Input: part model. Units: mm. Frame: model coordinates. Face numbers are marked on the shaded views. A direction names the side the tool comes from. Round coordinates to 2 decimals unless told otherwise and drop trailing zeros. Order: outer loops, then holes, each group sorted by start corner. A loop starts at its lowest first (then second) coordinate and runs counter-clockwise, first axis right, second up. Notation, with made-up numbers: (43, 40) -> (57, 40) arc R23 ccw to (57, 57) -> close; hole circle Ø9 at (68.5, -35.75). An arc over 180 degrees is marked (long way). Answer as CSV lines item,"result". Start each with the question number.
1) Section query B-B, the plane z = 43. Output: boundary loops of the cut face in (x, y), and give its area (3 significant figures).
2) Access query for the marked faces 1, 2 and 3. Directions: +Z, -Z, +X, -X, +Y, -Y. A direction counts if a zero-diameter tool reaches every point of the face in a straight line with its end or side. Return the directions, or none.
3) First-contact query: P1, Ø12, axis at x = 79, z = 30, coming from the +Y side; P2, Ø5, axis at y = 70.5, z = 21.5, coming from the +X side. Flat tips, straight axial feed; report the tip coordinate or a pass-through.
4) Line query: L1, parallel to X at y = 37, z = 7; L2, parallel to Y at x = 109.5, z = 47; L3, parallel to Y at x = 33, z = 33.5. Output: solid intervals per line, ascending.
5) Section query A-A, the plane x = 28.5. Output: boundary loops of the cut face in (y, z), and give its area (3 significant figures).
```python
from build123d import *

# Parameters (mm, degrees)
EXTRUDE_1_DEPTH     = 80
SKETCH_2_W          = 10
SKETCH_2_H          = 70
CUT_EXTRUDE_1_DEPTH = 250
SKETCH_3_W          = 70
SKETCH_3_H          = 10
CUT_EXTRUDE_2_DEPTH = 250
SKETCH_4_R          = 2.692710991
CUT_EXTRUDE_3_DEPTH = 10


with BuildPart() as part:
    # Эскиз1 → Бобышка-Вытянуть1 (new body)
    with BuildSketch(Plane.XY):
        Polygon((0, 0), (0, 220), (250, 220), (250, 140), (80, 140), (80, 0), align=None)
    extrude(amount=EXTRUDE_1_DEPTH)

    # Эскиз2 → Вырез-Вытянуть1 (cut)
    with BuildSketch(Plane.XZ):
        with Locations((5, 35)):
            Rectangle(SKETCH_2_W, SKETCH_2_H)
    extrude(amount=-CUT_EXTRUDE_1_DEPTH, mode=Mode.SUBTRACT)

    # Эскиз3 → Вырез-Вытянуть2 (cut)
    with BuildSketch(Plane(origin=(250, 0, 0), x_dir=(0, 0, -1), z_dir=(1, 0, 0))):
        with Locations((-35, 215)):
            Rectangle(SKETCH_3_W, SKETCH_3_H)
    extrude(amount=-CUT_EXTRUDE_2_DEPTH, mode=Mode.SUBTRACT)

    # Эскиз4 → Вырез-Вытянуть3 (cut)
    with BuildSketch(Plane.XY.offset(80)):
        with Locations((178.22144368, 213.38359115)):
            Circle(SKETCH_4_R)
    extrude(amount=-CUT_EXTRUDE_3_DEPTH, mode=Mode.SUBTRACT)


solid = part.part
```
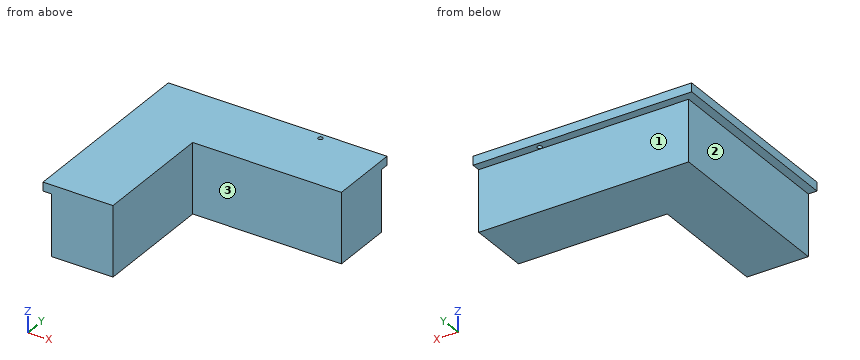
Findings:
1,outline,"(10, 0) -> (80, 0) -> (80, 140) -> (250, 140) -> (250, 210) -> (10, 210) -> close"
1,area,"26,600 mm^2"
2,face 1,"-Z, +X, -X, +Y"
2,face 2,"-Z, -X, +Y, -Y"
2,face 3,"+Z, -Z, +X, -Y"
3,P1,"stops at y = 210"
3,P2,"stops at x = 80"
4,L1,"x = 10 to 80"
4,L2,"y = 140 to 210"
4,L3,"y = 0 to 210"
5,outline,"(0, 0) -> (210, 0) -> (210, 70) -> (220, 70) -> (220, 80) -> (0, 80) -> close"
5,area,"16,900 mm^2"
